Geometry check sheet. Reference: the model listing, model coordinates, mm. A direction names the side the tool comes from. Give positions to 0.01 mm unless a question says otherwise; leave off trailing zeros. Write each loop counter-clockwise with the first axis right and the second up, starting at its lowest first coordinate (ties: lowest second). Pieces come first, ordered by that corner, then holes.
(1) Depth check by flat-ended pin: P1, Ø1.7, axis at x = -12.59, z = -4.58, coming from the -Y side; P2, Ø4, axis at x = 78.5, z = 4.5, coming from the +Y side; P3, Ø6.5, axis at x = -13, y = 8.5, coming from the -Z side; P4, Ø7.5, axis at x = 213, z = -3.5, coming from the +Y side. Enter the tip coordinate at first touch or a pass-through.
(2) Thickness scan on line 1 along Z through (x, y) = (120.5, 6.75); line 2 along X through (y, z) = (2.75, -1.5); line 3 along Y through (x, z) = (120.5, 24). Record the ranges inside material, lowest first.
(3) Cross-section at A-A (x = 141). Record the boundary of the cut face in (y, z), and give its area (3 significant figures).
(4) Cross-section at C-C (x = 88). Record the boundary of the cut face in (y, z).
(5) Tool access check on faces 1 (the cylindrical face through (72.475, 9.768, -1.901)), 2 (the flat face through (-12, 5, -3)), 3 (the flat face through (99, 4, -7.075)). Record the directions out of +Z, -Z, +X, -X, +Y, -Y that give a thin tool (end or side, any length) a straight path to the whole face; none if there is none.
(6) Cross-section at B-B (z = 13). Record the boundary of the cut face in (x, y), and give its area (3 significant figures).
(7) Cross-section at D-D (x = 37.5). Record the boundary of the cut face in (y, z), and give its area (3 significant figures).
(8) Mould release check, pull along Z, two halves, no side actions. Record for faces 4 (the cylindrical face through (26.583, 10.507, 20.774)), 5 (the flat face through (-13, 8, 1.925)), 6 (the flat face through (139.87, 6.03, 14.02)), 7 (the flat face through (-16.488, 5, 13)): +Z half, -Z half, draft (parallel to the pull), parting line (faces both ways), or undercut.
```python
from build123d import *

# Parameters (mm, degrees)
SKETCH_1_W           = 234.5
SKETCH_1_H           = 39.5
EXTRUDE_1_DEPTH      = 11
SKETCH_2_W           = 9
SKETCH_2_H           = 9
SKETCH_2_H_2         = 7
CUT_EXTRUDE_1_DEPTH  = 6
FILLET_2_R           = 2
SKETCH_3_R           = 1.4
CUT_EXTRUDE_2_DEPTH  = 6
FILLET_5_R           = 1
SKETCH_4_R           = 1.4
CUT_EXTRUDE_3_DEPTH  = 30
SKETCH_6_W           = 19.5
SKETCH_6_H           = 23.5
CUT_EXTRUDE_4_DEPTH  = 7.5
FILLET_7_R           = 2
SKETCH_7_W           = 37
SKETCH_7_H           = 13
CUT_EXTRUDE_5_DEPTH  = 7.5
CHAMFER_1_SIZE       = 10
CHAMFER_1_SIZE_2     = 7.812856265
SKETCH_8_R           = 1.4
CUT_EXTRUDE_6_DEPTH  = 37.5
CUT_EXTRUDE_8_DEPTH  = 2.5
SKETCH_10_R          = 1.75
CUT_EXTRUDE_9_DEPTH  = 13.5
SKETCH_11_W          = 52
SKETCH_11_H          = 48
CUT_EXTRUDE_10_DEPTH = 1
EXTRUDE_START        = 1
SKETCH_12_R          = 3
SKETCH_12_R_2        = 1.75
EXTRUDE_2_DEPTH      = 1
EXTRUDE_START_2      = 2.5
SKETCH_13_R          = 2.5
SKETCH_13_R_2        = 1.4
EXTRUDE_3_DEPTH      = 2.5
SKETCH_14_W          = 58.122310869
SKETCH_14_H          = 32.5
CUT_EXTRUDE_11_DEPTH = 1.5
EXTRUDE_START_3      = 1.5
SKETCH_15_R          = 2.75
SKETCH_15_R_2        = 1.4
EXTRUDE_4_DEPTH      = 1.5
CUT_EXTRUDE_12_DEPTH = 2.5


# Some blends are built 0.0001 mm under size
with BuildPart() as part:
    # 草图1 → 凸台-拉伸1 (new body)
    with BuildSketch(Plane(origin=(0, 0, 0), x_dir=(1, 0, 0), z_dir=(0, 1, 0))):
        with Locations((100.761595342, -12.674606198)):
            Rectangle(SKETCH_1_W, SKETCH_1_H)
    extrude(amount=EXTRUDE_1_DEPTH)

    # 草图2 → 切除-拉伸1 (cut)
    with BuildSketch(Plane(origin=(0, 11, 0), x_dir=(1, 0, 0), z_dir=(0, 1, 0))):
        with Locations((-11.988404658, 2.575393802)):
            Rectangle(SKETCH_2_W, SKETCH_2_H)
        with Locations((213.511595342, 3.575393802)):
            Rectangle(SKETCH_2_W, SKETCH_2_H_2)
    extrude(amount=-CUT_EXTRUDE_1_DEPTH, mode=Mode.SUBTRACT)

    # 圆角2
    fillet_2_edges = [part.edges().sort_by_distance(p)[0] for p in [
        (-7.488404658, 8, 1.924606198),
        (209.011595342, 8, -0.075393802),
    ]]
    fillet(fillet_2_edges, radius=FILLET_2_R)

    # 草图3 → 切除-拉伸2 (cut)
    with BuildSketch(Plane(origin=(0, 5, 0), x_dir=(1, 0, 0), z_dir=(0, 1, 0))):
        with Locations(Location((214.111595342, 4.575393802, 0), (0, 0, 270))):
            Circle(SKETCH_3_R)
        with Locations(Location((-12.588404658, 4.575393802, 0), (0, 0, 270))):
            Circle(SKETCH_3_R)
    extrude(amount=-CUT_EXTRUDE_2_DEPTH, mode=Mode.SUBTRACT)

    # 圆角5
    fillet_5_edges = [part.edges().sort_by_distance(p)[0] for p in [
        (-16.488404658, 2.5, -7.075393802),
        (218.011595342, 2.5, -7.075393802),
    ]]
    fillet(fillet_5_edges, radius=FILLET_5_R)

    # 草图4 → 切除-拉伸3 (cut)
    with BuildSketch(Plane(origin=(0, 11, 0), x_dir=(1, 0, 0), z_dir=(0, 1, 0))):
        with Locations(Location((206.011595342, -28.424606198, 0), (0, 0, 270))):
            Circle(SKETCH_4_R)
        with Locations(Location((173.511595342, -28.424606198, 0), (0, 0, 270))):
            Circle(SKETCH_4_R)
    extrude(amount=-CUT_EXTRUDE_3_DEPTH, mode=Mode.SUBTRACT)

    # 草图6 → 切除-拉伸4 (cut)
    with BuildSketch(Plane(origin=(0, 11, 0), x_dir=(1, 0, 0), z_dir=(0, 1, 0))):
        with Locations((208.261595342, -11.674606198)):
            Rectangle(SKETCH_6_W, SKETCH_6_H)
    extrude(amount=-CUT_EXTRUDE_4_DEPTH, mode=Mode.SUBTRACT)

    # 圆角7
    fillet_7_edges = [part.edges().sort_by_distance(p)[0] for p in [
        (211.011595342, 8, -0.075393802),
    ]]
    fillet(fillet_7_edges, radius=FILLET_7_R - 0.0001)  # a hair under: the kernel refuses the full size

    # 草图7 → 切除-拉伸5 (cut)
    with BuildSketch(Plane(origin=(0, 11, 0), x_dir=(1, 0, 0), z_dir=(0, 1, 0))):
        with Locations((162.011595342, -13.924606198)):
            Rectangle(SKETCH_7_W, SKETCH_7_H)
    extrude(amount=-CUT_EXTRUDE_5_DEPTH, mode=Mode.SUBTRACT)

    # 倒角1
    # the kernel refuses this chamfer: 10, 7.812856265 mm, written as the material it takes off along each edge
    with BuildSketch(Plane(origin=(143.511595342, 11, 20.424606198), x_dir=(-0.9997151392093143, 0.023867141339117017, 0), z_dir=(0, 0, -1))) as chamfer_1_piece_1_section:
        Polygon((CHAMFER_1_SIZE * 0.999715139209, -CHAMFER_1_SIZE * 0.0238671413391), (-CHAMFER_1_SIZE_2 * 0.0238671413393, -CHAMFER_1_SIZE_2 * 0.999715139218), (0, 0), align=None)
    chamfer_1_piece_1 = extrude(amount=13, mode=Mode.PRIVATE)
    chamfer_1_piece_1 = split(chamfer_1_piece_1, bisect_by=Plane(origin=(140.173122789, 3.5, 13.924606198), z_dir=(0, 1, 0)), keep=Keep.TOP, mode=Mode.PRIVATE)
    add(chamfer_1_piece_1, mode=Mode.SUBTRACT)

    # 草图8 → 切除-拉伸6 (cut)
    with BuildSketch(Plane(origin=(0, 11, 0), x_dir=(1, 0, 0), z_dir=(0, 1, 0))):
        with Locations(Location((120.511595342, -26.924606198, 0), (0, 0, 270))):
            Circle(SKETCH_8_R)
        with Locations(Location((69.99674604, 1.575393802, 0), (0, 0, 270))):
            Circle(SKETCH_8_R)
    extrude(amount=-CUT_EXTRUDE_6_DEPTH, mode=Mode.SUBTRACT)

    # 草图9 → 切除-拉伸8 (cut)
    with BuildSketch(Plane(origin=(0, 11, 0), x_dir=(1, 0, 0), z_dir=(0, 1, 0))):
        Polygon((51.103694557, 8.790142976), (123.268586448, -31.924606198), (150.036795822, 15.520729333), (77.871903931, 56.235478507), align=None)
    extrude(amount=-CUT_EXTRUDE_8_DEPTH, mode=Mode.SUBTRACT)

    # 草图10 → 切除-拉伸9 (cut)
    with BuildSketch(Plane(origin=(0, 11, 0), x_dir=(1, 0, 0), z_dir=(0, 1, 0))):
        with Locations(Location((13.511595342, -21.424606198, 0), (0, 0, 270))):
            Circle(SKETCH_10_R)
        with Locations(Location((29.511595342, -21.424606198, 0), (0, 0, 270))):
            Circle(SKETCH_10_R)
    extrude(amount=-CUT_EXTRUDE_9_DEPTH, mode=Mode.SUBTRACT)

    # 草图11 → 切除-拉伸10 (cut)
    with BuildSketch(Plane(origin=(0, 11, 0), x_dir=(1, 0, 0), z_dir=(0, 1, 0))):
        with Locations((21.511595342, -8.424606198)):
            Rectangle(SKETCH_11_W, SKETCH_11_H)
    extrude(amount=-CUT_EXTRUDE_10_DEPTH, mode=Mode.SUBTRACT)

    # 草图12 → 凸台-拉伸2 (add)
    # profile 1 of 2: a face of its own
    with BuildSketch(Plane(origin=(0, 10, 0), x_dir=(1, 0, 0), z_dir=(0, 1, 0)).offset(EXTRUDE_START)):
        with Locations(Location((13.511595342, -21.424606198, 0), (0, 0, 270))):
            Circle(SKETCH_12_R)
        with Locations(Location((13.511595342, -21.424606198, 0), (0, 0, 270))):
            Circle(SKETCH_12_R_2, mode=Mode.SUBTRACT)
    # profile 2 of 2: a face of its own
    with BuildSketch(Plane(origin=(0, 10, 0), x_dir=(1, 0, 0), z_dir=(0, 1, 0)).offset(EXTRUDE_START)):
        with Locations(Location((29.511595342, -21.424606198, 0), (0, 0, 270))):
            Circle(SKETCH_12_R)
        with Locations(Location((29.511595342, -21.424606198, 0), (0, 0, 270))):
            Circle(SKETCH_12_R_2, mode=Mode.SUBTRACT)
    extrude(amount=-EXTRUDE_2_DEPTH)

    # 草图13 → 凸台-拉伸3 (add)
    # profile 1 of 2: a face of its own
    with BuildSketch(Plane(origin=(0, 8.5, 0), x_dir=(1, 0, 0), z_dir=(0, 1, 0)).offset(EXTRUDE_START_2)):
        with Locations(Location((69.99674604, 1.575393802, 0), (0, 0, 270))):
            Circle(SKETCH_13_R)
        with Locations(Location((69.99674604, 1.575393802, 0), (0, 0, 270))):
            Circle(SKETCH_13_R_2, mode=Mode.SUBTRACT)
    # profile 2 of 2: a face of its own
    with BuildSketch(Plane(origin=(0, 8.5, 0), x_dir=(1, 0, 0), z_dir=(0, 1, 0)).offset(EXTRUDE_START_2)):
        with Locations(Location((120.511595342, -26.924606198, 0), (0, 0, 270))):
            Circle(SKETCH_13_R)
        with Locations(Location((120.511595342, -26.924606198, 0), (0, 0, 270))):
            Circle(SKETCH_13_R_2, mode=Mode.SUBTRACT)
    extrude(amount=-EXTRUDE_3_DEPTH)

    # 草图14 → 切除-拉伸11 (cut)
    with BuildSketch(Plane(origin=(0, 11, 0), x_dir=(1, 0, 0), z_dir=(0, 1, 0))):
        with Locations((188.950439908, -16.174606198)):
            Rectangle(SKETCH_14_W, SKETCH_14_H)
    extrude(amount=-CUT_EXTRUDE_11_DEPTH, mode=Mode.SUBTRACT)

    # 草图15 → 凸台-拉伸4 (add)
    # profile 1 of 2: a face of its own
    with BuildSketch(Plane(origin=(0, 9.5, 0), x_dir=(1, 0, 0), z_dir=(0, 1, 0)).offset(EXTRUDE_START_3)):
        with Locations(Location((173.511595342, -28.424606198, 0), (0, 0, 270))):
            Circle(SKETCH_15_R)
        with Locations(Location((173.511595342, -28.424606198, 0), (0, 0, 270))):
            Circle(SKETCH_15_R_2, mode=Mode.SUBTRACT)
    # profile 2 of 2: a face of its own
    with BuildSketch(Plane(origin=(0, 9.5, 0), x_dir=(1, 0, 0), z_dir=(0, 1, 0)).offset(EXTRUDE_START_3)):
        with Locations(Location((206.011595342, -28.424606198, 0), (0, 0, 270))):
            Circle(SKETCH_15_R)
        with Locations(Location((206.011595342, -28.424606198, 0), (0, 0, 270))):
            Circle(SKETCH_15_R_2, mode=Mode.SUBTRACT)
    extrude(amount=-EXTRUDE_4_DEPTH)

    # 草图16 → 切除-拉伸12 (cut)
    with BuildSketch(Plane(origin=(0, 11, 0), x_dir=(1, 0, 0), z_dir=(0, 1, 0))):
        Polygon((123.268586448, -31.924606198), (146.066616294, -31.924606198), (168.070047273, 7.075393802), (145.272017426, 7.075393802), align=None)
    extrude(amount=-CUT_EXTRUDE_12_DEPTH, mode=Mode.SUBTRACT)


solid = part.part
```
Reply:
1. P1: passes through
1. P2: stops at y = 11
1. P3: stops at z = 1.92
1. P4: stops at y = 5
2. line 1: z = -7.08 to 25.52, 28.32 to 32.42
2. line 2: x = -16.49 to 68.6, 71.39 to 218.01
2. line 3: y = 0 to 8.5
3. outline: (0, -7.08) - (8.5, -7.08) - (8.5, 7.42) - (5.15, 7.42) - (5.15, 20.42) - (8.5, 20.42) - (8.5, 31.92) - (11, 31.92) - (11, 32.42) - (0, 32.42) - close
3. area: 293 mm2
4. outline: (0, -7.08) - (8.5, -7.08) - (8.5, 12.03) - (11, 12.03) - (11, 32.42) - (0, 32.42) - close
5. face 1: +Y
5. face 2: -Z, -X, +Y
5. face 3: -Z, +X, -X, +Y, -Y
6. outline: (-16.49, 0) - (218.01, 0) - (218.01, 3.5) - (198.51, 3.5) - (198.51, 9.5) - (180.51, 9.5) - (180.51, 3.5) - (143.11, 3.5) - (136.71, 8.5) - (89.73, 8.5) - (89.73, 11) - (47.51, 11) - (47.51, 10) - (-4.49, 10) - (-4.49, 11) - (-16.49, 11) - close
6. area: 1,920 mm2
7. outline: (0, -7.08) - (10, -7.08) - (10, 32.42) - (0, 32.42) - close
7. area: 395 mm2
8. face 4: parting line
8. face 5: -Z half
8. face 6: undercut
8. face 7: draft
